from build123d import *

# Parameters (mm, degrees)
SKETCH_W        = 180
SKETCH_H        = 110
PAD_DEPTH       = 130
THICKNESS_T     = -2.5
CHAMFER_SIZE    = 8
SKETCH001_R     = 1.25
HOLE001_DEPTH   = 16
HOLE001_TIPS_R  = 1.25
HOLE_DEPTH      = 15
HOLE_TIPS_R     = 1.25
SKETCH002_W     = 178.2
SKETCH002_H     = 108.2
POCKET_DEPTH    = 4
FILLET_R        = 0.15
POCKET001_DEPTH = 1
SKETCH004_R     = 1
POCKET002_DEPTH = 3
SKETCH005_R     = 4.5
SKETCH005_R_2   = 3.5
SKETCH005_R_3   = 6
POCKET003_DEPTH = 5
SKETCH007_R     = 1.75
SKETCH007_R_2   = 3.5
POCKET004_DEPTH = 5
SKETCH009_R     = 1.75
SKETCH009_R_2   = 4.75
SKETCH009_R_3   = 3.35
SKETCH009_W     = 71
SKETCH009_H     = 44
POCKET005_DEPTH = 5


with BuildPart() as part:
    # Sketch → Pad (new body)
    with BuildSketch(Plane.XY):
        Rectangle(SKETCH_W, SKETCH_H)
    extrude(amount=PAD_DEPTH)

    # Thickness
    thickness_openings = [part.faces().sort_by_distance(p)[0] for p in [
        (0, 0, 130),
    ]]
    offset(amount=THICKNESS_T, openings=thickness_openings, kind=Kind.INTERSECTION)

    # Chamfer
    chamfer_edges = [part.edges().sort_by_distance(p)[0] for p in [
        (-87.5, 52.5, 66.25),
        (-87.5, -52.5, 66.25),
        (87.5, 52.5, 66.25),
        (87.5, -52.5, 66.25),
    ]]
    chamfer(chamfer_edges, length=CHAMFER_SIZE)

    # Sketch001 (on Face1 of Chamfer) → Hole001 (cut)
    with BuildSketch(Plane.XY.offset(130)):
        with Locations((-86, 51)):
            Circle(SKETCH001_R)
        with Locations((86, 51)):
            Circle(SKETCH001_R)
        with Locations((86, -51)):
            Circle(SKETCH001_R)
        with Locations((-86, -51)):
            Circle(SKETCH001_R)
    extrude(amount=-HOLE001_DEPTH, mode=Mode.SUBTRACT)

    # Hole001 tips → Hole001 tip 1 section 0
    with BuildSketch(Plane.XY.offset(114), mode=Mode.PRIVATE) as hole001_tip_1_s0:
        with Locations((-86, 51)):
            Circle(HOLE001_TIPS_R)
    loft([hole001_tip_1_s0.sketch, Vertex(-86, 51, 113.248924)], mode=Mode.SUBTRACT)

    # Hole001 tips → Hole001 tip 2 section 0
    with BuildSketch(Plane.XY.offset(114), mode=Mode.PRIVATE) as hole001_tip_2_s0:
        with Locations((86, 51)):
            Circle(HOLE001_TIPS_R)
    loft([hole001_tip_2_s0.sketch, Vertex(86, 51, 113.248924)], mode=Mode.SUBTRACT)

    # Hole001 tips → Hole001 tip 3 section 0
    with BuildSketch(Plane.XY.offset(114), mode=Mode.PRIVATE) as hole001_tip_3_s0:
        with Locations((86, -51)):
            Circle(HOLE001_TIPS_R)
    loft([hole001_tip_3_s0.sketch, Vertex(86, -51, 113.248924)], mode=Mode.SUBTRACT)

    # Hole001 tips → Hole001 tip 4 section 0
    with BuildSketch(Plane.XY.offset(114), mode=Mode.PRIVATE) as hole001_tip_4_s0:
        with Locations((-86, -51)):
            Circle(HOLE001_TIPS_R)
    loft([hole001_tip_4_s0.sketch, Vertex(-86, -51, 113.248924)], mode=Mode.SUBTRACT)

    # Sketch001 (on Face1 of Chamfer) → Hole (cut)
    with BuildSketch(Plane.XY.offset(130)):
        with Locations((-86, 51)):
            Circle(SKETCH001_R)
        with Locations((86, 51)):
            Circle(SKETCH001_R)
        with Locations((86, -51)):
            Circle(SKETCH001_R)
        with Locations((-86, -51)):
            Circle(SKETCH001_R)
    extrude(amount=-HOLE_DEPTH, mode=Mode.SUBTRACT)

    # Hole tips → Hole tip 1 section 0
    with BuildSketch(Plane.XY.offset(115), mode=Mode.PRIVATE) as hole_tip_1_s0:
        with Locations((-86, 51)):
            Circle(HOLE_TIPS_R)
    loft([hole_tip_1_s0.sketch, Vertex(-86, 51, 114.248924)], mode=Mode.SUBTRACT)

    # Hole tips → Hole tip 2 section 0
    with BuildSketch(Plane.XY.offset(115), mode=Mode.PRIVATE) as hole_tip_2_s0:
        with Locations((86, 51)):
            Circle(HOLE_TIPS_R)
    loft([hole_tip_2_s0.sketch, Vertex(86, 51, 114.248924)], mode=Mode.SUBTRACT)

    # Hole tips → Hole tip 3 section 0
    with BuildSketch(Plane.XY.offset(115), mode=Mode.PRIVATE) as hole_tip_3_s0:
        with Locations((86, -51)):
            Circle(HOLE_TIPS_R)
    loft([hole_tip_3_s0.sketch, Vertex(86, -51, 114.248924)], mode=Mode.SUBTRACT)

    # Hole tips → Hole tip 4 section 0
    with BuildSketch(Plane.XY.offset(115), mode=Mode.PRIVATE) as hole_tip_4_s0:
        with Locations((-86, -51)):
            Circle(HOLE_TIPS_R)
    loft([hole_tip_4_s0.sketch, Vertex(-86, -51, 114.248924)], mode=Mode.SUBTRACT)

    # Sketch002 (on Face9 of Hole) → Pocket (cut)
    with BuildSketch(Plane.XY.offset(130)):
        Rectangle(SKETCH002_W, SKETCH002_H)
    extrude(amount=-POCKET_DEPTH, mode=Mode.SUBTRACT)

    # Fillet
    fillet_edges = [part.edges().sort_by_distance(p)[0] for p in [
        (90, -55, 65),
        (90, 55, 65),
        (-90, -55, 65),
        (-90, 55, 65),
    ]]
    fillet(fillet_edges, radius=FILLET_R)

    # Sketch003 (on Face14 of Fillet) → Pocket001 (cut)
    with BuildSketch(Plane(origin=(0, 0, 0), x_dir=(1, 0, 0), z_dir=(0, 0, -1))):
        Polygon((0, 0), (12.5, 15), (17.5, 15), (17.5, -20), (12.5, -20), (12.5, 7), (2.5, -5), (-2.5, -5), (-12.5, 7), (-12.5, -20), (-17.5, -20), (-17.5, 15), (-12.5, 15), align=None)
    extrude(amount=-POCKET001_DEPTH, mode=Mode.SUBTRACT)

    # Sketch004 (on Face41 of Pocket001) → Pocket002 (cut)
    with BuildSketch(Plane(origin=(0, 0, 1), x_dir=(1, 0, 0), z_dir=(0, 0, -1))):
        with Locations((-15, 11.5)):
            Circle(SKETCH004_R)
        with Locations((-11.5, 9)):
            Circle(SKETCH004_R)
        with Locations((-9.1, 6.25)):
            Circle(SKETCH004_R)
        with Locations((-15, 8)):
            Circle(SKETCH004_R)
        with Locations((-15, 4.5)):
            Circle(SKETCH004_R)
        with Locations((-15, 1)):
            Circle(SKETCH004_R)
        with Locations((-15, -2.5)):
            Circle(SKETCH004_R)
        with Locations((-15, -6)):
            Circle(SKETCH004_R)
        with Locations((-15, -9.5)):
            Circle(SKETCH004_R)
        with Locations((-15, -13)):
            Circle(SKETCH004_R)
        with Locations((-15, -16.5)):
            Circle(SKETCH004_R)
        with Locations((-6.7, 3.5)):
            Circle(SKETCH004_R)
        with Locations((-4.3, 0.75)):
            Circle(SKETCH004_R)
        with Locations((-1.9, -2)):
            Circle(SKETCH004_R)
        with Locations((1.9, -2)):
            Circle(SKETCH004_R)
        with Locations((4.3, 0.75)):
            Circle(SKETCH004_R)
        with Locations((6.7, 3.5)):
            Circle(SKETCH004_R)
        with Locations((11.5, 9)):
            Circle(SKETCH004_R)
        with Locations((15, 11.5)):
            Circle(SKETCH004_R)
        with Locations((9.1, 6.25)):
            Circle(SKETCH004_R)
        with Locations((15, 8)):
            Circle(SKETCH004_R)
        with Locations((15, 4.5)):
            Circle(SKETCH004_R)
        with Locations((15, 1)):
            Circle(SKETCH004_R)
        with Locations((15, -2.5)):
            Circle(SKETCH004_R)
        with Locations((15, -6)):
            Circle(SKETCH004_R)
        with Locations((15, -9.5)):
            Circle(SKETCH004_R)
        with Locations((15, -16.5)):
            Circle(SKETCH004_R)
        with Locations((15, -13)):
            Circle(SKETCH004_R)
    extrude(amount=-POCKET002_DEPTH, mode=Mode.SUBTRACT)

    # Sketch005 (on Face6 of Pocket002) → Pocket003 (cut)
    with BuildSketch(Plane.YZ.offset(90)):
        with Locations((34.85, 116.5)):
            Circle(SKETCH005_R)
        with Locations((14.85, 116.5)):
            Circle(SKETCH005_R_2)
        with Locations((-29.85, 116.5)):
            Circle(SKETCH005_R_3)
    extrude(amount=-POCKET003_DEPTH, mode=Mode.SUBTRACT)

    # Sketch007 (on Face6 of Pocket003) → Pocket004 (cut)
    with BuildSketch(Plane.YZ.offset(90)):
        with Locations((27.65, 13)):
            Circle(SKETCH007_R)
        with Locations((27.65, 97.5)):
            Circle(SKETCH007_R)
        with Locations((-37.35, 97.5)):
            Circle(SKETCH007_R)
        with Locations((-37.35, 13)):
            Circle(SKETCH007_R)
        with Locations((-13.85, 24)):
            Circle(SKETCH007_R_2)
        with Locations((-13.85, 41.5)):
            Circle(SKETCH007_R_2)
        with Locations((-13.85, 61.5)):
            Circle(SKETCH007_R_2)
    extrude(amount=-POCKET004_DEPTH, mode=Mode.SUBTRACT)

    # Sketch009 (on Face2 of Pocket004) → Pocket005 (cut)
    with BuildSketch(Plane(origin=(0, 55, 0), x_dir=(-1, 0, 0), z_dir=(0, 1, 0))):
        with Locations((72.25, 29.9)):
            Circle(SKETCH009_R)
        with Locations((-41.95, 29.9)):
            Circle(SKETCH009_R)
        with Locations((-41.95, 104.1)):
            Circle(SKETCH009_R)
        with Locations((72.25, 104.1)):
            Circle(SKETCH009_R)
        with Locations((54.15, 103)):
            Circle(SKETCH009_R_2)
        with Locations((39.15, 103)):
            Circle(SKETCH009_R_2)
        with Locations((24.15, 103)):
            Circle(SKETCH009_R_2)
        with Locations((9.15, 103)):
            Circle(SKETCH009_R_2)
        with Locations((54.15, 87)):
            Circle(SKETCH009_R_3)
        with Locations((39.15, 87)):
            Circle(SKETCH009_R_3)
        with Locations((24.15, 87)):
            Circle(SKETCH009_R_3)
        with Locations((9.15, 87)):
            Circle(SKETCH009_R_3)
        with Locations((64.15, 85)):
            Circle(SKETCH009_R_2)
        with Locations((32.65, 49)):
            Rectangle(SKETCH009_W, SKETCH009_H)
    extrude(amount=-POCKET005_DEPTH, mode=Mode.SUBTRACT)


solid = part.part
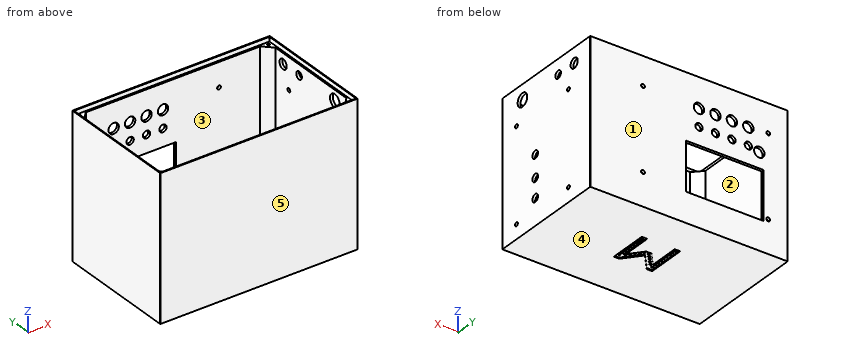
Model file for the job. Use its own axes, mm. Face numbers are marked on the shaded views. A direction names the side the tool comes from. Round coordinates to 2 decimals unless told otherwise and drop trailing zeros. Loops run counter-clockwise (first coordinate to the right, second up) from the corner with the lowest first, then second, coordinate; pieces in that order, holes last. Notation, with made-up numbers: (53, 24) -> (106, 24) arc R22 ccw to (106, 31) -> close; hole circle Ø10 at (69, -0.5). An arc over 180 degrees is marked (long way). Answer as CSV lines item,"result". Start each with the question number.
1) Slice it at A-A (z = 77). List the corners of the cut face in (x, y).
2) Tool access for the marked faces 1 and 2: list every direction of +Z, -Z, +X, -X, +Y, -Y with a clear straight run to the whole face (end or side of a thin tool).
3) Mould opens along Y. For the marked faces 3, 4 and 5 say: +Y half, -Y half, draft (parallel to the pull), parting line (faces both ways), or undercut.
4) Slice it at D-D (z = 53.5). List the corners of the cut face in (x, y).
5) Pin check, flat tips, straight feed: P1, Ø2, axis at x = 86, y = 51, coming from the +Z side; P2, Ø3, axis at x = -15, y = -1, coming from the +Z side; P3, Ø2.5, axis at x = -4.3, y = -0.75, coming from the -Z side; P4, Ø2, axis at x = -57, y = -35.5, coming from the -Z side. Stop position of each tip, or through.
6) Slice it at C-C (x = 67). List the corners of the cut face in (y, z).
7) Slice it at B-B (x = -24.15). List the corners of the cut face in (y, z), plus the area to 3 significant figures.
8) Probe line 1 along Z through (x, y) = (-9, 53); line 2 along Z through (x, y) = (88.4, -37.35); line 3 along X through (y, z) = (17.5, 89). List the from-to ranges inside material, lowest first.
Filled in:
1,outline,"(-90, -54.85) arc R0.15 ccw to (-89.85, -55) -> (89.85, -55) arc R0.15 ccw to (90, -54.85) -> (90, 54.85) arc R0.15 ccw to (89.85, 55) -> (-89.85, 55) arc R0.15 ccw to (-90, 54.85) -> close; hole (-87.5, -44.5) -> (-79.5, -52.5) -> (79.5, -52.5) -> (87.5, -44.5) -> (87.5, 44.5) -> (79.5, 52.5) -> (-79.5, 52.5) -> (-87.5, 44.5) -> close"
2,face 1,"+Z, -Z, +X, -X, +Y"
2,face 2,"+Z"
3,face 3,"undercut"
3,face 4,"draft"
3,face 5,"-Y half"
4,outline,"(-90, -54.85) arc R0.15 ccw to (-89.85, -55) -> (89.85, -55) arc R0.15 ccw to (90, -54.85) -> (90, 54.85) arc R0.15 ccw to (89.85, 55) -> (2.85, 55) -> (2.85, 52.5) -> (79.5, 52.5) -> (87.5, 44.5) -> (87.5, -44.5) -> (79.5, -52.5) -> (-79.5, -52.5) -> (-87.5, -44.5) -> (-87.5, 44.5) -> (-79.5, 52.5) -> (-68.15, 52.5) -> (-68.15, 55) -> (-89.85, 55) arc R0.15 ccw to (-90, 54.85) -> close"
5,P1,"stops at z = 113.85"
5,P2,"stops at z = 2.5"
5,P3,"stops at z = 1"
5,P4,"stops at z = 0"
6,outline,"(-55, 0) -> (55, 0) -> (55, 130) -> (54.1, 130) -> (54.1, 126) -> (52.5, 126) -> (52.5, 2.5) -> (-52.5, 2.5) -> (-52.5, 126) -> (-54.1, 126) -> (-54.1, 130) -> (-55, 130) -> close"
7,outline,"(-55, 0) -> (55, 0) -> (55, 27) -> (52.5, 27) -> (52.5, 2.5) -> (-52.5, 2.5) -> (-52.5, 126) -> (-54.1, 126) -> (-54.1, 130) -> (-55, 130) -> close; (52.5, 71) -> (55, 71) -> (55, 83.65) -> (52.5, 83.65) -> close; (52.5, 90.35) -> (55, 90.35) -> (55, 98.25) -> (52.5, 98.25) -> close; (52.5, 107.75) -> (55, 107.75) -> (55, 130) -> (54.1, 130) -> (54.1, 126) -> (52.5, 126) -> close"
7,area,"749 mm2"
8,line 1,"z = 0 to 27, 71 to 83.65, 90.35 to 98.25, 107.75 to 126"
8,line 2,"z = 0 to 11.25, 14.75 to 95.75, 99.25 to 126"
8,line 3,"x = -90 to -87.5, 87.5 to 90"
